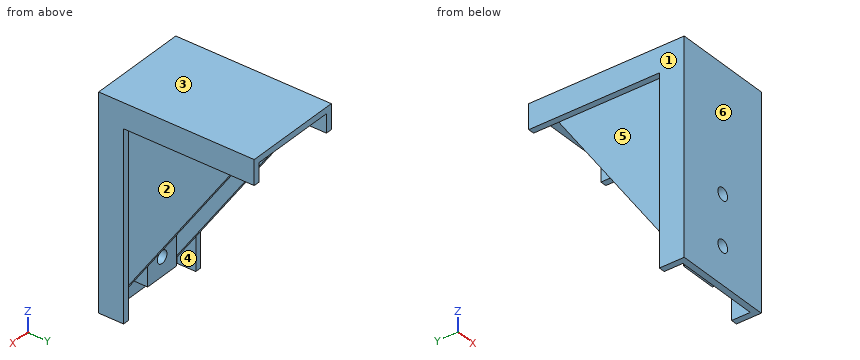
from build123d import *

# Parameters (mm, degrees)
BOSS_EXTRUDE1_DEPTH     = 31.25
BOSS_EXTRUDE2_DEPTH     = 41.25
BOSS_EXTRUDE3_DEPTH     = 1.25
SKETCH6_W               = 7.5
SKETCH6_H               = 22.5
SKETCH6_R               = 1.25
BOSS_EXTRUDE4_DEPTH     = 3.75
CUT_EXTRUDE1_DEPTH      = 53.974050251
CUT_EXTRUDE1_DEPTH_BACK = 53.974050251
SKETCH6_2_R             = 1.25


with BuildPart() as part:
    # Sketch1 → Boss-Extrude1 (new body)
    with BuildSketch(Plane(origin=(0, 0, 0), x_dir=(1, 0, 0), z_dir=(0, 1, 0))):
        Polygon((-10, 0), (10, 0), (10, 5), (8.75, 5), (8.75, 1.25), (-8.75, 1.25), (-8.75, 5), (-10, 5), align=None)
    extrude(amount=BOSS_EXTRUDE1_DEPTH)

    # Sketch2 → Boss-Extrude2 (add)
    with BuildSketch(Plane(origin=(0, 0, -1.25), x_dir=(-1, 0, 0), z_dir=(0, 0, -1))):
        Polygon((-10, 5), (-10, 0), (10, 0), (10, 5), (8.75, 5), (8.75, 1.25), (-8.75, 1.25), (-8.75, 5), align=None)
    extrude(amount=BOSS_EXTRUDE2_DEPTH)

    # Sketch4 → Boss-Extrude3 (add)
    with BuildSketch(Plane(origin=(7.5, 0, 0), x_dir=(0, 0, -1), z_dir=(1, 0, 0))):
        Polygon((1.25, 28.75), (1.25, 1.25), (41.25, 1.25), align=None)
    boss_extrude3 = extrude(amount=BOSS_EXTRUDE3_DEPTH)

    # Mirror1: Boss-Extrude3 across plane
    add(boss_extrude3.mirror(Plane(origin=(0, 0, 0), x_dir=(0, 0, 1), z_dir=(1, 0, 0))))

    # Sketch6 → Boss-Extrude4 (add)
    with BuildSketch(Plane(origin=(0, 1.25, 0), x_dir=(1, 0, 0), z_dir=(0, 1, 0))):
        with Locations((0, 27.5)):
            Rectangle(SKETCH6_W, SKETCH6_H)
        with Locations(Location((0, 35, 0), (0, 0, 180))):
            Circle(SKETCH6_R, mode=Mode.SUBTRACT)
        with Locations(Location((0, 25, 0), (0, 0, 180))):
            Circle(SKETCH6_R, mode=Mode.SUBTRACT)
    extrude(amount=BOSS_EXTRUDE4_DEPTH)

    # Sketch6_2 → Cut-Extrude1 (cut, two sides: drawn at the far end of the back side and taken through both)
    with BuildSketch(Plane(origin=(0, 1.25, 0), x_dir=(1, 0, 0), z_dir=(0, 1, 0)).offset(-CUT_EXTRUDE1_DEPTH_BACK)):
        with Locations(Location((0, 35, 0), (0, 0, 180))):
            Circle(SKETCH6_2_R)
        with Locations(Location((0, 25, 0), (0, 0, 180))):
            Circle(SKETCH6_2_R)
    extrude(amount=CUT_EXTRUDE1_DEPTH + CUT_EXTRUDE1_DEPTH_BACK, mode=Mode.SUBTRACT)


solid = part.part
Could you check a few things on this model? Use its own coordinates, in mm. Face numbers are marked on the shaded views. A direction names the side the tool comes from. Give positions to 0.01 mm unless a question says otherwise; leave off trailing zeros. Order: outer loops, then holes, each group sorted by start corner. A loop starts at its lowest first (then second) coordinate and runs counter-clockwise, first axis right, second up.
Item 1: I'm going to push flat-ended pins straight in: pin 1 (2 mm diameter, centred on x = 0, z = -35, fed in from +Y); pin 2 (14 mm diameter, centred on y = 12.5, z = -19, fed in from -X); pin 3 (5 mm diameter, centred on x = 1, y = 13, fed in from -Z); pin 4 (5 mm diameter, centred on x = 2, z = -29, fed in from +Y). Where does each tip first touch, or does it pass through?
Item 2: If we section it at C-C, the plane y = 5.5: Write out the boundary of the cut face in (x, z), plus the area to 3 significant figures.
Item 3: I need wall thicknesses on line 1 (X direction, y = 1.4, z = -25); line 2 (Z direction, x = 0, y = 2.6); line 3 (X direction, y = 4, z = -37). Which ranges of each line are inside material? Lowest first, please.
Item 4: For the marked faces 5 and 6, which set-ups out of +Z, -Z, +X, -X, +Y, -Y let a thin tool reach every point of the face, with its end or its side?
Item 5: If we mould it in two halves opening along X, with no side actions, what happens to the marked faces 1, 2, 3 and 4? For each: pulls with the +X half, pulls with the -X half, needs draft (parallel to the pull), parting line crosses it, or undercut.
Item 6: If we section it at D-D, the plane x = 5: Write out the boundary of the cut face in (y, z), plus the area to 3 significant figures.
Item 7: If we section it at A-A, the plane x = 0: Write out the boundary of the cut face in (y, z).
Item 8: If we section it at B-B, the plane z = -34.5: Write out the boundary of the cut face in (x, y), plus the area to 3 significant figures.
Values:
1. pin 1: passes through
1. pin 2: stops at x = -8.75
1. pin 3: stops at z = -1.25
1. pin 4: stops at y = 5
2. outline: (-10, -5) - (-8.75, -5) - (-8.75, -35.07) - (-7.5, -35.07) - (-7.5, -1.25) - (7.5, -1.25) - (7.5, -35.07) - (8.75, -35.07) - (8.75, -5) - (10, -5) - (10, 0) - (-10, 0) - close
2. area: 119 mm2
3. line 1: x = -10 to -7.5, -3.75 to -1.25, 1.25 to 3.75, 7.5 to 10
3. line 2: z = -38.75 to -36.25, -33.75 to -26.25, -23.75 to -16.25, -1.25 to 0
3. line 3: x = -10 to -7.5, -3.75 to 3.75, 7.5 to 10
4. face 5: -Z, -X, +Y
4. face 6: +Z, -Z, +X, -X, -Y
5. face 1: pulls with the -X half
5. face 2: pulls with the +X half
5. face 3: needs draft
5. face 4: undercut
6. outline: (0, -42.5) - (1.25, -42.5) - (1.25, -1.25) - (31.25, -1.25) - (31.25, 0) - (0, 0) - close
6. area: 90.6 mm2
7. outline: (0, -42.5) - (1.25, -42.5) - (1.25, -38.75) - (5, -38.75) - (5, -36.25) - (0, -36.25) - close; (0, -33.75) - (5, -33.75) - (5, -26.25) - (0, -26.25) - close; (0, -23.75) - (5, -23.75) - (5, -16.25) - (1.25, -16.25) - (1.25, -1.25) - (31.25, -1.25) - (31.25, 0) - (0, 0) - close
8. outline: (-10, 0) - (-1.15, 0) - (-1.15, 5) - (-3.75, 5) - (-3.75, 1.25) - (-7.5, 1.25) - (-7.5, 5.89) - (-8.75, 5.89) - (-8.75, 5) - (-10, 5) - close; (1.15, 0) - (10, 0) - (10, 5) - (8.75, 5) - (8.75, 5.89) - (7.5, 5.89) - (7.5, 1.25) - (3.75, 1.25) - (3.75, 5) - (1.15, 5) - close
8. area: 62.6 mm2
